Verification items for the finished model (mm, model axes). A direction names the side the tool comes from. Give positions to 0.01 mm unless a question says otherwise; leave off trailing zeros. Loops run counter-clockwise (first coordinate to the right, second up) from the corner with the lowest first, then second, coordinate; pieces in that order, holes last. Notation, with made-up numbers: (-15, 87) -> (35, 87) arc R20 cw to (35, 97) -> close; hole circle Ø10 at (-21, 43.25). An arc over 180 degrees is marked (long way). Answer in a Markdown table with one row per item. Add a question column.
Q1. Material ranges on probe 1 along Y at (x, z) = (0, 3.9); probe 2 along Y at (x, z) = (0, 2.9); probe 3 along X at (y, z) = (2.75, 1.25), recorded low to high.
Q2. Release check for a two-part mould opening along Y. For faces 1 (the face through (-1.46, -6.59, 3.51)), 2 (the face through (1, 3, 0)), 3 (the face through (2, -4, 3.8)) record: pulls with the +Y half, pulls with the -Y half, needs draft (parallel to the pull), parting line crosses it, or undercut.
Q3. Set-up check for faces 4 (the face through (-5, -4, 3)), 5 (the face through (-5, -2, 0)): record each of +Z, -Z, +X, -X, +Y, -Y from which the full face is reachable in a straight line by a thin tool's end or side.
Q4. Section check D-D on z = 3.25. Enter the section's corners in (x, y), and give its area (3 significant figures).
Q5. Section check C-C on z = 1.65. Enter the section's corners in (x, y), and give its area (3 significant figures).
Q6. Gauge pin test, flat ends, axial feed: P1, Ø1, axis at x = 4, z = 2, coming from the +Y side; P2, Ø1, axis at x = -3, z = 1.5, coming from the -Y side; P3, Ø6, axis at x = 2.5, y = -0.5, coming from the +Z side; P4, Ø1, axis at y = 0.5, z = 2, coming from the -X side. Record the tip position at first contact, or that the pin passes through.
```python
from build123d import *

# Parameters (mm, degrees)
SKETCH_1_R          = 6
EXTRUDE_1_DEPTH     = 4
SKETCH_2_R          = 6.75
EXTRUDE_2_DEPTH     = 1
SKETCH_3_R          = 3
CUT_EXTRUDE_1_DEPTH = 5
SKETCH_4_R          = 5
SKETCH_4_R_2        = 4
CUT_EXTRUDE_2_DEPTH = 0.2
SKETCH_5_R          = 5.75
SKETCH_5_R_2        = 4
CUT_EXTRUDE_3_DEPTH = 0.2
FILLET_1_R          = 0.1


with BuildPart() as part:
    # 草圖1 → 填料-伸長1 (new body)
    with BuildSketch(Plane.XY):
        Circle(SKETCH_1_R)
    extrude(amount=EXTRUDE_1_DEPTH)

    # 草圖2 → 填料-伸長2 (add)
    with BuildSketch(Plane.XY.offset(4)):
        Circle(SKETCH_2_R)
    extrude(amount=-EXTRUDE_2_DEPTH)

    # 草圖3 → 除料-伸長1 (cut, through all)
    with BuildSketch(Plane(origin=(0, 0, 0), x_dir=(-1, 0, 0), z_dir=(0, 0, -1))):
        Circle(SKETCH_3_R)
    extrude(amount=-CUT_EXTRUDE_1_DEPTH, mode=Mode.SUBTRACT)

    # 草圖4 → 除料-伸長2 (cut)
    with BuildSketch(Plane(origin=(0, 0, 0), x_dir=(-1, 0, 0), z_dir=(0, 0, -1))):
        Circle(SKETCH_4_R)
        Circle(SKETCH_4_R_2, mode=Mode.SUBTRACT)
    extrude(amount=-CUT_EXTRUDE_2_DEPTH, mode=Mode.SUBTRACT)

    # 草圖5 → 除料-伸長3 (cut)
    with BuildSketch(Plane.XY.offset(4)):
        Circle(SKETCH_5_R)
        Circle(SKETCH_5_R_2, mode=Mode.SUBTRACT)
    extrude(amount=-CUT_EXTRUDE_3_DEPTH, mode=Mode.SUBTRACT)

    # 圓角1
    fillet_1_edges = [part.edges().sort_by_distance(p)[0] for p in [
        (-6, 0, 0),
    ]]
    fillet(fillet_1_edges, radius=FILLET_1_R)


solid = part.part
```
Taken from the geometry:
| question | item | result |
|---|---|---|
| 1 | probe 1 | y = -6.75 to -5.75, -4 to -3, 3 to 4, 5.75 to 6.75 |
| 1 | probe 2 | y = -6 to -3, 3 to 6 |
| 1 | probe 3 | x = -5.33 to -1.2, 1.2 to 5.33 |
| 2 | face 1 | parting line crosses it |
| 2 | face 2 | needs draft |
| 2 | face 3 | undercut |
| 3 | face 4 | -Z |
| 3 | face 5 | -Z, +X, -X, +Y, -Y |
| 4 | outline | circle Ø13.5 at (0, 0); hole circle Ø6 at (0, 0) |
| 4 | area | 115 mm² |
| 5 | outline | circle Ø12 at (0, 0); hole circle Ø6 at (0, 0) |
| 5 | area | 84.8 mm² |
| 6 | P1 | stops at y = 4.87 |
| 6 | P2 | stops at y = -5.45 |
| 6 | P3 | stops at z = 4 |
| 6 | P4 | stops at x = -6 |
